from build123d import *

# Parameters (mm, degrees)
F0_W     = 50
F0_H     = 50
F1_DEPTH = 256
F2_W     = 1100
F2_H     = 500
F3_DEPTH = 50


with BuildPart() as f1:
    # F0 (on Top) → F1 (new body)
    with BuildSketch(Plane.XY):
        with Locations((25, -25)):
            Rectangle(F0_W, F0_H)
    extrude(amount=F1_DEPTH)



with BuildPart() as f1b:
    # F0 (on Top) → F1, piece 2 (new body)
    with BuildSketch(Plane.XY):
        with Locations((25, 525)):
            Rectangle(F0_W, F0_H)
    extrude(amount=F1_DEPTH)


with BuildPart() as f1c:
    # F0 (on Top) → F1, piece 3 (new body)
    with BuildSketch(Plane.XY):
        with Locations((1175, -25)):
            Rectangle(F0_W, F0_H)
    extrude(amount=F1_DEPTH)


with BuildPart() as f1d:
    # F0 (on Top) → F1, piece 4 (new body)
    with BuildSketch(Plane.XY):
        with Locations((1175, 525)):
            Rectangle(F0_W, F0_H)
    extrude(amount=F1_DEPTH)


with BuildPart() as f1_1:
    add(f1.part)

    add(f1b.part)  # F3 merges F1b

    add(f1c.part)  # F3 merges F1c

    add(f1d.part)  # F3 merges F1d
    # F2 (on face) → F3 (join)
    with BuildSketch(Plane.XY.offset(256)):
        Polygon((0, 0), (0, -50), (50, -50), (1150, -50), (1200, -50), (1200, 0), (1200, 500), (1200, 550), (1150, 550), (50, 550), (0, 550), (0, 500), align=None)
        with Locations((600, 250)):
            Rectangle(F2_W, F2_H, mode=Mode.SUBTRACT)
    extrude(amount=F3_DEPTH)


solid = f1_1.part
Work out the finished part from the listing and answer in its coordinate system (mm). A direction names the side the tool comes from. Coordinates: 2 decimals unless noted, no trailing zeros. Loops run counter-clockwise (first coordinate to the right, second up) from the corner with the lowest first, then second, coordinate; pieces in that order, holes last. Notation, with made-up numbers: M 21,45 L 27,45 A24 ccw 27,55 Z; hole C 52.5,51 d1. An arc over 180 degrees is marked long. Answer in a Markdown table with one row per item. Add a question column.
1. Consider L1, parallel to X at y = -20.5, z = 208.5; L2, parallel to Y at x = 1006, z = 283. Determine where each line is inside the solid, lowest interval first.
2. Flat-ended cylindrical pins translate along their axes: P1, Ø15, axis at y = -31.5, z = 153, coming from the -X side; P2, Ø25, axis at x = 1174.5, y = 276.5, coming from the -Z side. Find the tip coordinate at first contact, or state that the pin passes through.
3. A tool of negligible diameter and unlimited length cuts with its end or side. For faces 1 (the flat face through (25, 500, 126)), 2 (the flat face through (553, -15, 306)), 3 (the flat face through (592, 0, 281)), 4 (the flat face through (1150, -25, 126)), 5 (the flat face through (1175, -25, 0)), from which of +Z, -Z, +X, -X, +Y, -Y can it reach the whole face along a straight path? Write none if from no direction.
4. Find section A-A, the plane x = 599.5. Write down the section's boundary in (y, z), then the cut area to 3 significant figures.
5. Find section B-B, the plane z = 26. Write down the section's boundary in (x, y).
6. The mould has two halves that part along Y. Classify faces 6 (the flat face through (25, 254, 256)), 7 (the flat face through (592, 500, 281)), 8 (the flat face through (0, 229, 266)), 9 (the flat face through (597, -50, 277)): pulls with the +Y half, pulls with the -Y half, needs draft (parallel to the pull), parting line crosses it, or undercut.
7. Find section C-C, the plane y = 470. Write down the section's boundary in (x, z), then the cut area to 3 significant figures.
Reported:
| question | item | result |
|---|---|---|
| 1 | L1 | x = 0 to 50, 1150 to 1200 |
| 1 | L2 | y = -50 to 0, 500 to 550 |
| 2 | P1 | stops at x = 0 |
| 2 | P2 | stops at z = 256 |
| 3 | face 1 | -Z, +X, -X |
| 3 | face 2 | +Z, +X, -X, +Y, -Y |
| 3 | face 3 | +Z, -Z |
| 3 | face 4 | -Z, +Y, -Y |
| 3 | face 5 | -Z, +X, -X, +Y, -Y |
| 4 | outline | M -50,256 L 0,256 L 0,306 L -50,306 Z; M 500,256 L 550,256 L 550,306 L 500,306 Z |
| 4 | area | 5,000 mm^2 |
| 5 | outline | M 0,-50 L 50,-50 L 50,0 L 0,0 Z; M 0,500 L 50,500 L 50,550 L 0,550 Z; M 1150,-50 L 1200,-50 L 1200,0 L 1150,0 Z; M 1150,500 L 1200,500 L 1200,550 L 1150,550 Z |
| 6 | face 6 | undercut |
| 6 | face 7 | undercut |
| 6 | face 8 | needs draft |
| 6 | face 9 | pulls with the -Y half |
| 7 | outline | M 0,256 L 50,256 L 50,306 L 0,306 Z; M 1150,256 L 1200,256 L 1200,306 L 1150,306 Z |
| 7 | area | 5,000 mm^2 |
